Read the model definition and answer for the solid it produces. Units are mm, in the model's axes. A direction names the side the tool comes from. Give positions to 0.01 mm unless a question says otherwise; leave off trailing zeros. Loops run counter-clockwise (first coordinate to the right, second up) from the corner with the lowest first, then second, coordinate; pieces in that order, holes last. Notation, with made-up numbers: (71, -28.5) - (115, -28.5) arc R27 cw to (115, -7.5) - close; hole circle Ø2 at (-39.75, 8.25). An arc over 180 degrees is marked (long way). Use a Markdown table: item, result. Add a question column.
Item 1: A cutting plane is placed at B-B (x = 33). Determine the outline of the cut face in (y, z).
Item 2: Which of the six approach directions +Z, -Z, +X, -X, +Y, -Y give full straight-line access (tool end or side, diameter ignored) to faces 4 (the face through (15.97, 6.53, 40.49)), 5 (the face through (0, 4, 45)), 6 (the face through (-27.5, 5, 1)), 7 (the face through (-45, -1, 1))?
Item 3: Consider probe 1 along X at (y, z) = (2.25, 37); probe 2 along Z at (x, y) = (-17, -1). Determine where each line is inside the solid, lowest interval first. Write a range as [from, to].
Item 4: A cutting plane is placed at D-D (x = -3.5). Determine the outline of the cut face in (y, z).
Item 5: A cutting plane is placed at C-C (y = 5.75). Determine the outline of the cut face in (x, z), plus the area to 3 significant figures.
Item 6: For a pull along X with two mould halves and no side action, classify faces 1 (the face through (-22, 4.5, 2)), 2 (the face through (38, 2, -1)), 3 (the face through (27.5, 5, 1)) as +X half, -X half, draft (parallel to the pull), parting line (faces both ways), or undercut.
Item 7: A cutting plane is placed at A-A (z = -23). Determine the outline of the cut face in (x, y), plus the area to 3 significant figures.
Item 8: Each of these flat-tipped pins is pushed along its axis until it touches: P1, Ø0.8, axis at y = 3, z = 13, coming from the -X side; P2, Ø15, axis at x = -15.5, z = 10, coming from the -Y side; P3, Ø3, axis at x = 32, z = 29.5, coming from the +Y side. Where does it stop, or does it pass through?
from build123d import *

# Parameters (mm, degrees)
SKETCH1_W           = 96
SKETCH1_H           = 96
SKETCH1_W_2         = 90
SKETCH1_H_2         = 90
BOSS_EXTRUDE1_DEPTH = 2
SKETCH1_3_W         = 96
SKETCH1_3_H         = 96
SKETCH1_3_W_2       = 90
SKETCH1_3_H_2       = 90
BOSS_EXTRUDE2_DEPTH = 3
BOSS_EXTRUDE3_DEPTH = 96
SKETCH3_3_W         = 40.5
SKETCH3_3_H         = 4
BOSS_EXTRUDE4_DEPTH = 3
FILLET1_R           = 15


with BuildPart() as part:
    # Sketch1 → Boss-Extrude1 (new body)
    # profile 1 of 2: a face of its own
    with BuildSketch(Plane(origin=(0, 0, 0), x_dir=(1, 0, 0), z_dir=(0, 1, 0))):
        Rectangle(SKETCH1_W, SKETCH1_H)
        Rectangle(SKETCH1_W_2, SKETCH1_H_2, mode=Mode.SUBTRACT)
    # profile 2 of 2: a face of its own
    with BuildSketch(Plane(origin=(0, 0, 0), x_dir=(1, 0, 0), z_dir=(0, 1, 0))):
        Rectangle(SKETCH1_W_2, SKETCH1_H_2)
    extrude(amount=BOSS_EXTRUDE1_DEPTH)

    # Sketch1<3> → Boss-Extrude2 (add)
    with BuildSketch(Plane(origin=(0, 0, 0), x_dir=(1, 0, 0), z_dir=(0, 1, 0))):
        Rectangle(SKETCH1_3_W, SKETCH1_3_H)
        Rectangle(SKETCH1_3_W_2, SKETCH1_3_H_2, mode=Mode.SUBTRACT)
    extrude(amount=-BOSS_EXTRUDE2_DEPTH)

    # Sketch3 → Boss-Extrude3 (add)
    with BuildSketch(Plane.XY.offset(48)):
        Polygon((-27.5, 8.5), (-27.5, 2), (-24.25, 2), (-24.25, 4.5), (-20.25, 4.5), (-20.25, 8.5), align=None)
        Polygon((24.25, 4.5), (24.25, 2), (27.5, 2), (27.5, 8.5), (20.25, 8.5), (20.25, 4.5), align=None)
    extrude(amount=-BOSS_EXTRUDE3_DEPTH)

    # Sketch3<3> → Boss-Extrude4 (add)
    with BuildSketch(Plane.XY.offset(48)):
        Polygon((-24.25, 4.5), (-24.25, 2), (24.25, 2), (24.25, 4.5), (20.25, 4.5), (-20.25, 4.5), align=None)
        with Locations((0, 6.5)):
            Rectangle(SKETCH3_3_W, SKETCH3_3_H)
    extrude(amount=-BOSS_EXTRUDE4_DEPTH)

    # Fillet1
    fillet1_edges = [part.edges().sort_by_distance(p)[0] for p in [
        (-20.25, 6.5, 45),
        (20.25, 6.5, 45),
    ]]
    fillet(fillet1_edges, radius=FILLET1_R)


solid = part.part
Geometry says:
| question | item | result |
|---|---|---|
| 1 | outline | (-3, -48) - (2, -48) - (2, 48) - (-3, 48) - (-3, 45) - (0, 45) - (0, -45) - (-3, -45) - close |
| 2 | face 4 | -Z, +Y |
| 2 | face 5 | -Z |
| 2 | face 6 | +Z, -Z, -X, +Y |
| 2 | face 7 | -Y |
| 3 | probe 1 | [-27.5, -24.25], [24.25, 27.5] |
| 3 | probe 2 | [-48, -45], [45, 48] |
| 4 | outline | (-3, -48) - (2, -48) - (2, 45) - (8.5, 45) - (8.5, 48) - (-3, 48) - (-3, 45) - (0, 45) - (0, -45) - (-3, -45) - close |
| 5 | outline | (-27.5, -48) - (-20.25, -48) - (-20.25, 30) arc R15 cw to (-5.25, 45) - (5.25, 45) arc R15 cw to (20.25, 30) - (20.25, -48) - (27.5, -48) - (27.5, 48) - (-27.5, 48) - close |
| 5 | area | 1,610 mm² |
| 6 | face 1 | undercut |
| 6 | face 2 | draft |
| 6 | face 3 | +X half |
| 7 | outline | (-48, -3) - (-45, -3) - (-45, 0) - (45, 0) - (45, -3) - (48, -3) - (48, 2) - (27.5, 2) - (27.5, 8.5) - (20.25, 8.5) - (20.25, 4.5) - (24.25, 4.5) - (24.25, 2) - (-24.25, 2) - (-24.25, 4.5) - (-20.25, 4.5) - (-20.25, 8.5) - (-27.5, 8.5) - (-27.5, 2) - (-48, 2) - close |
| 7 | area | 284 mm² |
| 8 | P1 | x = -27.5 |
| 8 | P2 | y = 0 |
| 8 | P3 | y = 2 |
